from build123d import *

# Parameters (mm, degrees)
F0_W         = 3.175
F0_H         = 38.1
F3_R         = 3.175
F4_W         = 3.175
F4_H         = 55.6163180947
F5_DEPTH     = 30.734
F6_W         = 3.175
F6_H         = 64.323036778
F7_DEPTH     = 27.178
F8_R         = 11.5282463958
F9_DEPTH     = 72.136
F10_T2_ANGLE = 359.64
F10_T4_ANGLE = 359.64
F10_T6_ANGLE = 359.64
F10_T8_ANGLE = 359.64


# Not quite as in the source:
# - a fillet or chamfer that OpenCascade refuses, or shapes differently, is made with other operations: its cross-section is extruded or revolved along the edge and cut away or added


with BuildPart() as f2:
    # F0 (on Front) → F2 (revolve)
    with BuildSketch(Plane.XZ):
        Polygon((7.1327639744, 64.2934367061), (23.8125, 0), (23.8125, 3.5723163746), (25.5098140885, 3.5723163746), (9.5913732515, 64.9312771426), align=None)
        Polygon((23.8125, 3.5723163746), (23.8125, 0), (50.8, 0), (50.8, 3.5723163746), (47.625, 3.5723163746), (25.5098140885, 3.5723163746), align=None)
        with Locations((49.2125, 22.6223163746)):
            Rectangle(F0_W, F0_H)
    revolve(axis=Axis((0, 0, 38.2007025182), (0, 0, 1)))

    # F3
    f3_edges = [f2.edges().sort_by_distance(p)[0] for p in [
        (-50.8, 0, 0),
        (-23.8125, 0, 0),
        (-25.509814, 0, 3.572316),
        (-47.625, 0, 3.572316),
    ]]
    fillet(f3_edges, radius=F3_R)

    # F4 (on Front) → F5 (cut, symmetric)
    with BuildSketch(Plane.XZ):
        with Locations((1.5875, 40.5081590474)):
            Rectangle(F4_W, F4_H)
        Polygon((-3.175, 12.7), (0, 12.7), (0, 68.3163180947), (0, 68.3765411377), (-3.175, 68.3765411377), align=None)
    extrude(amount=F5_DEPTH, both=True, mode=Mode.SUBTRACT)

    # F6 (on Right) → F7 (cut, symmetric)
    with BuildSketch(Plane.YZ):
        Polygon((0, 77.023036778), (0, 12.7), (3.175, 12.7), (3.175, 80.2117586136), (0, 80.2117586136), align=None)
        with Locations((-1.5875, 44.861518389)):
            Rectangle(F6_W, F6_H)
    extrude(amount=F7_DEPTH, both=True, mode=Mode.SUBTRACT)

    # F8 (on Top) → F9 (cut)
    with BuildSketch(Plane.XY):
        Circle(F8_R)
    extrude(amount=F9_DEPTH, mode=Mode.SUBTRACT)

    # F10: chamfer of 10.16 x 33.02 on 4 edges, made by hand

    # F10_s1 → F10_t2 (revolve, cut)
    with BuildSketch(Plane(origin=(0, 0, 0), x_dir=(0, 0, 1), z_dir=(-0.7093247296, -0.7048818539, 0))):
        Polygon((15.3887617085, 19.8201720703), (57.5106823112, 11.5282463958), (47.3506823112, 11.5282463958), align=None)
    revolve(axis=Axis((0, 0, 47.3506823112), (0, 0, -1)), revolution_arc=F10_T2_ANGLE, mode=Mode.SUBTRACT)

    # F10_s3 → F10_t4 (revolve, cut)
    with BuildSketch(Plane(origin=(0, 0, 0), x_dir=(0, 0, 1), z_dir=(-0.7048818539, 0.7093247296, 0))):
        Polygon((15.3887617085, 19.8201720703), (57.5106823112, 11.5282463958), (47.3506823112, 11.5282463958), align=None)
    revolve(axis=Axis((0, 0, 47.3506823112), (0, 0, -1)), revolution_arc=F10_T4_ANGLE, mode=Mode.SUBTRACT)

    # F10_s5 → F10_t6 (revolve, cut)
    with BuildSketch(Plane(origin=(0, 0, 0), x_dir=(0, 0, 1), z_dir=(0.7093247296, 0.7048818539, 0))):
        Polygon((15.3887617085, 19.8201720703), (57.5106823112, 11.5282463958), (47.3506823112, 11.5282463958), align=None)
    revolve(axis=Axis((0, 0, 47.3506823112), (0, 0, -1)), revolution_arc=F10_T6_ANGLE, mode=Mode.SUBTRACT)

    # F10_s7 → F10_t8 (revolve, cut)
    with BuildSketch(Plane(origin=(0, 0, 0), x_dir=(0, 0, 1), z_dir=(0.7048818539, -0.7093247296, 0))):
        Polygon((15.3887617085, 19.8201720703), (57.5106823112, 11.5282463958), (47.3506823112, 11.5282463958), align=None)
    revolve(axis=Axis((0, 0, 47.3506823112), (0, 0, -1)), revolution_arc=F10_T8_ANGLE, mode=Mode.SUBTRACT)


solid = f2.part
Verification items for the finished model (mm, model axes). A direction names the side the tool comes from. Coordinates: 2 decimals unless noted, no trailing zeros. Order: outer loops, then holes, each group sorted by start corner. A loop starts at its lowest first (then second) coordinate and runs counter-clockwise, first axis right, second up. Notation, with made-up numbers: M -33,81.25 L 23,81.25 A25 cw 23,102.25 Z; hole C -11,12 d6. An arc over 180 degrees is marked long. One line per item, written item: value. Start each with the question number.
Item 1: Sectioned sample at D-D on z = 33. Record the cut outline in (x, y) (3 decimals), then the cut area to 3 significant figures.
Item 2: Depth check by flat-ended pin: P1, Ø1.5, axis at x = 27.5, z = 8.5, coming from the +Y side; P2, Ø3, axis at x = -1.5, y = 21, coming from the +Z side; P3, Ø8, axis at y = 38.5, z = 33.5, coming from the +X side; P4, Ø5, axis at x = 37.5, y = 38, coming from the +Z side. Enter the tip coordinate at first touch or a pass-through.
Item 3: Sectioned sample at C-C on z = 53. Record the cut outline in (x, y) (3 decimals).
Item 4: Mould release check, pull along X, two halves, no side actions. Record for faces 3 (the cylindrical face through (-37.794, -28.979, 24.454)), 4 (the flat face through (-20, -20, 0)): pulls with the +X half, pulls with the -X half, needs draft (parallel to the pull), parting line crosses it, or undercut.
Item 5: Sectioned sample at A-A on z = 22.5. Record the cut outline in (x, y) (3 decimals), then the cut area to 3 significant figures.
Item 6: Sectioned sample at B-B on y = 0. Record the cut outline in (x, z) (3 decimals).
Item 7: Thickness scan on probe 1 along Y at (x, z) = (0, 19.5) (3 decimals); probe 2 along Y at (x, z) = (-18, 11.5); probe 3 along X at (y, z) = (-9.5, 26.5). Record the ranges inside material, lowest first.
Item 8: Access from +Z, -Z, +X, -X, +Y, -Y to the whole of each face (thin tool, end or side, straight path). Record for faces 1 (the flat face through (0, 22, 12.7)), 2 (the conical face through (11.15, -10.96, 36.65)).
Calculated:
1. outline: C 0,0 d101.6; M -17.591,-3.175 A17.875 ccw -3.175,-17.591 L -3.175,-16.042 A16.353 cw -16.042,-3.175 Z; M -17.591,3.175 L -16.042,3.175 A16.353 cw -3.175,16.042 L -3.175,17.591 A17.875 ccw Z; M 3.175,-17.591 A17.875 ccw 17.591,-3.175 L 16.042,-3.175 A16.353 cw 3.175,-16.042 Z; M 3.175,16.042 A16.353 cw 16.042,3.175 L 17.591,3.175 A17.875 ccw 3.175,17.591 Z; hole C 0,0 d95.25
1. area: 1,110 mm^2
2. P1: y = 43.19
2. P2: z = 12.7
2. P3: x = 37.29
2. P4: through
3. outline: M -12.283,-3.175 A12.687 ccw -3.175,-12.283 L -3.175,-12.003 A12.416 cw -12.003,-3.175 Z; M -12.283,3.175 L -12.003,3.175 A12.416 cw -3.175,12.003 L -3.175,12.283 A12.687 ccw Z; M 3.175,-12.283 A12.687 ccw 12.283,-3.175 L 12.003,-3.175 A12.416 cw 3.175,-12.003 Z; M 3.175,12.003 A12.416 cw 12.003,3.175 L 12.283,3.175 A12.687 ccw 3.175,12.283 Z
4. face 3: undercut
4. face 4: needs draft
5. outline: C 0,0 d101.6; M -20.353,-3.175 A20.599 ccw -3.175,-20.353 L -3.175,-18.145 A18.42 cw -18.145,-3.175 Z; M -20.353,3.175 L -18.145,3.175 A18.42 cw -3.175,18.145 L -3.175,20.353 A20.599 ccw Z; M 3.175,-20.353 A20.599 ccw 20.353,-3.175 L 18.145,-3.175 A18.42 cw 3.175,-18.145 Z; M 3.175,18.145 A18.42 cw 18.145,3.175 L 20.353,3.175 A20.599 ccw 3.175,20.353 Z; hole C 0,0 d95.25
5. area: 1,190 mm^2
6. outline: M -50.8,3.175 A3.175 ccw -47.625,0 L -26.269,0 A3.175 ccw -23.196,2.378 L -20.518,12.7 L -23.142,12.7 L -24.893,5.95 A3.175 cw -27.966,3.572 L -44.45,3.572 A3.175 cw -47.625,6.747 L -47.625,41.672 L -50.8,41.672 Z; M 20.518,12.7 L 23.196,2.378 A3.175 ccw 26.269,0 L 47.625,0 A3.175 ccw 50.8,3.175 L 50.8,41.672 L 47.625,41.672 L 47.625,6.747 A3.175 cw 44.45,3.572 L 27.966,3.572 A3.175 cw 24.893,5.95 L 23.142,12.7 Z
7. probe 1: -50.8 to -47.625, 47.625 to 50.8
7. probe 2: -47.5 to -44.09, -15.03 to -10.48, 10.48 to 15.03, 44.09 to 47.5
7. probe 3: -49.9 to -46.67, -17.1 to -14.85, 14.85 to 17.1, 46.67 to 49.9
8. face 1: +Z
8. face 2: -Z
